Autodesk Inventor part; units mm, degrees
ref_plane "YZ Plane" through (0, 0, 0) normal (1, 0, 0) x (0, 1, 0)
ref_plane "XZ Plane" through (0, 0, 0) normal (0, 1, 0) x (-1, 0, 0)
ref_plane "XY Plane" through (0, 0, 0) normal (0, 0, 1) x (1, 0, 0)
sketch "Sketch1" plane through (0, 0, 0) normal (0, 0, 1) x (1, 0, 0)
  line L0 (-50, -100) -> (50, -100)
  line L1 (50, -100) -> (50, 100)
  line L2 (50, 100) -> (-50, 100)
  line L3 (-50, 100) -> (-50, -100)
  line L4 (-50, -100) -> (50, 100) construction
  line L5 (50, -100) -> (-50, 100) construction
  point P0 (0, 0)
  dimension "d0" = 100
  dimension "d1" = 200
extrude "Extrusion1" add sketch "Sketch1" along normal blind 5
sketch "Sketch2" plane through (-50, 100, 0) normal (0, 1, 0) x (1, 0, 0)
  line L0 (0, 0) -> (100, 0)
  line L1 (0, 0) -> (49.9986, 49.9986)
  line L2 (49.9986, 49.9986) -> (53.5341, 46.463)
  line L3 (53.5341, 46.463) -> (3.5355, -3.5355)
  line L4 (3.5355, -3.5355) -> (0, 0)
  line L5 (0, 0) -> (70.7086, 0) construction
  line L6 (100.108, -0.1109) -> (53.5341, 46.463)
  line L7 (53.5341, 46.463) -> (49.9986, 42.9275)
  line L8 (49.9986, 42.9275) -> (96.5724, -3.6464)
  line L9 (96.5724, -3.6464) -> (100.108, -0.1109)
  point P0 (50, 0)
  point P1 (49.9986, 42.9275)
  dimension "d4" = 45
  dimension "d5" = 5
  dimension "d6" = 5
extrude "Extrusion2" add sketch "Sketch2" against normal blind 30 contours L1 L2 L3 L0 | L0 L3 L4 | L8 L3 L6 L0 | L0 L6 L9 L8
sketch "Sketch6" plane through (0, 0, 5) normal (0, 0, 1) x (1, 0, 0)
  line L0 (4.9986, 75) -> (-5.0014, 75)
  line L1 (-25.0014, 55) -> (-25.0014, 45)
  line L2 (-5.0014, 25) -> (4.9986, 25)
  line L3 (24.9986, 45) -> (24.9986, 55)
  line L4 (24.9986, 75) -> (-25.0014, 25) construction
  line L5 (-25.0014, 75) -> (24.9986, 25) construction
  arc A0 (4.9986, 25) -> (24.9986, 45) centre (4.9986, 45) ccw
  arc A1 (24.9986, 55) -> (4.9986, 75) centre (4.9986, 55) ccw
  arc A2 (-5.0014, 75) -> (-25.0014, 55) centre (-5.0014, 55) ccw
  arc A3 (-25.0014, 45) -> (-5.0014, 25) centre (-5.0014, 45) ccw
  point P0 (0, 0)
  point P1 (-0.0014, 50)
  dimension "d21" = 50
  dimension "d22" = 50
  dimension "d23" = 20
extrude "Extrusion6" cut sketch "Sketch6" against normal blind 5
sketch "Sketch10" plane through (-50, 100, 5) normal (0, 1, 0) x (1, 0, 0)
  line L0 (0, 5) -> (7.0711, 5)
  line L1 (49.9986, 54.9986) -> (99.9971, 5)
  line L2 (0, 5) -> (49.9986, 54.9986)
  line L3 (49.9986, 54.9986) -> (46.463, 58.5341)
  line L4 (46.463, 58.5341) -> (-3.5355, 8.5355)
  line L5 (-3.5355, 8.5355) -> (0, 5)
  line L6 (100, 4.7812) -> (100, 0)
  line L7 (100, 4.7812) -> (49.9986, 54.9986)
  line L8 (49.9986, 54.9986) -> (53.5417, 58.5265)
  line L9 (53.5417, 58.5265) -> (103.5431, 8.3091)
  line L10 (103.5431, 8.3091) -> (100, 4.7812)
  line L11 (92.926, 5) -> (49.9986, 47.9275)
  line L12 (100, 0) -> (0, 0)
  line L13 (0, 0) -> (100, 0)
  point P0 (50, 5)
  dimension "d33" = 5
  dimension "d34" = 5
extrude "Extrusion9" add sketch "Sketch10" against normal blind 3
properties part number "fixation_v09"
Read the model definition and answer for the solid it produces. Units are mm, in the model's axes. A direction names the side the tool comes from. Round coordinates to 2 decimals unless told otherwise and drop trailing zeros. Write each loop counter-clockwise with the first axis right and the second up, starting at its lowest first coordinate (ties: lowest second). Pieces come first, ordered by that corner, then holes. Notation, with made-up numbers: (22.25, -24) - (39.25, -24) arc R15 cw to (39.25, -6) - close; hole circle Ø3 at (13.25, 22). An arc over 180 degrees is marked (long way). Use a Markdown table: item, result.
(1) Straight lines are drawn through the part: line 1 along Y through (x, z) = (-4, -41); line 2 along Y through (x, z) = (16.5, -36); line 3 along Z through (x, y) = (41, -47.5). For each, find the intervals that lie inside material, in ascending order. Write a range as [from, to].
Reported:
| item | result |
|---|---|
| line 1 | [70, 100] |
| line 2 | [97, 100] |
| line 3 | [0, 5] |
(2) The part is cut by section D-D (y = 39). Write down the section's boundary in (x, z), then the cut area to 3 significant figures.
Reported:
| item | result |
|---|---|
| outline | (-50, 0) - (-24.08, 0) - (-24.08, 5) - (-50, 5) - close; (24.08, 0) - (50, 0) - (50, 5) - (24.08, 5) - close |
| area | 259 mm2 |
(3) Which of the six approach directions +Z, -Z, +X, -X, +Y, -Y give full straight-line access (tool end or side, diameter ignored) to faces 4 (the flat face through (-21.165, 85.21, -21.764)), 5 (the cylindrical face through (-19.298, 31.014, 2.535)), 6 (the flat face through (1.75, 98.52, -51.74)), 7 (the cylindrical face through (-18.987, 69.297, 2.535)), 8 (the flat face through (-11, 70, -33))?
Reported:
| item | result |
|---|---|
| face 4 | +Y, -Y |
| face 5 | +Z, -Z |
| face 6 | -Z, +Y, -Y |
| face 7 | +Z |
| face 8 | -Z, +X, -X, -Y |
(4) The part is cut by section C-C (z = -20). Write down the section's boundary in (x, y).
Reported:
| item | result |
|---|---|
| outline | (-37.07, 97) - (-30, 97) - (-30, 70) - (-22.93, 70) - (-22.93, 100) - (-37.07, 100) - close; (22.93, 70) - (30, 70) - (30, 97) - (36.92, 97) - (36.92, 100) - (22.93, 100) - close |
(5) The part is cut by section B-B (x = -10.5). Write down the section's boundary in (y, z), then the cut area to 3 significant figures.
Reported:
| item | result |
|---|---|
| outline | (-100, 0) - (25.77, 0) - (25.77, 5) - (-100, 5) - close; (70, -39.5) - (97, -39.5) - (97, -46.57) - (100, -46.57) - (100, -32.43) - (70, -32.43) - close; (74.23, 0) - (100, 0) - (100, 5) - (74.23, 5) - close |
| area | 991 mm2 |
(6) Each of these flat-tipped pins is pushed along its axis until it touches: pin 1 Ø5.5 at (y, z) = (52.5, 2) entering from +X; pin 2 Ø1.5 at (x, y) = (21, -26.5) entering from -Z; pin 3 Ø15 at (x, z) = (23.5, -25) entering from -Y. Where does it stop, or does it pass through?
Reported:
| item | result |
|---|---|
| pin 1 | x = 50 |
| pin 2 | z = 0 |
| pin 3 | y = 70 |
(7) The mould has two halves that part along Y. Classify faces 1 (the flat face through (27, 97, -27)), 2 (the flat face through (-50, 1, 2)), 3 (the cylindrical face through (19.295, 68.986, 2.535)): released by +Y, released by -Y, zero draft, split by the parting line, or undercut.
Reported:
| item | result |
|---|---|
| face 1 | released by -Y |
| face 2 | zero draft |
| face 3 | undercut |
